from build123d import *

# Parameters (mm, degrees)
SKETCH_1_W                = 20
SKETCH_1_H                = 34
EXTRUDE_1_DEPTH           = 5
SKETCH_2_W                = 20
SKETCH_2_H                = 3
EXTRUDE_2_DEPTH           = 5
EXTRUDE_3_DEPTH           = 5
FILLET_1_R                = 3
CUT_EXTRUDE_1_DEPTH       = 2
SKETCH_7_R                = 1.6
CUT_EXTRUDE_2_DEPTH       = 41.087864079
SKETCH_8_R                = 1.75
CUT_EXTRUDE_3_DEPTH       = 41.087864079
CUT_EXTRUDE_5_DEPTH       = 3.2
SKETCH_14_W               = 10
SKETCH_14_H               = 3
EXTRUDE_26_DEPTH          = 51
SKETCH_11_W               = 51
SKETCH_11_H               = 87.152977717
SKETCH_11_R               = 11.1
SKETCH_11_R_2             = 1.6
EXTRUDE_27_DEPTH          = 5
CUT_EXTRUDE_7_DEPTH       = 3
SKETCH_16_R               = 1.6
CUT_EXTRUDE_8_DEPTH       = 89.921313531
EXTRUDE_28_DEPTH          = 6.7
SKETCH_18_W               = 40
SKETCH_18_H               = 5
CUT_EXTRUDE_9_DEPTH       = 5
CHAMFER_1_SIZE            = 2
SKETCH_19_W               = 1.7
SKETCH_19_H               = 23
EXTRUDE_31_DEPTH          = 5
SKETCH_20_W               = 5
SKETCH_20_H               = 28
EXTRUDE_33_DEPTH          = 5
EXTRUDE_34_DEPTH          = 1.7
SKETCH_24_R               = 11.1
CUT_EXTRUDE_10_DEPTH      = 1
CUT_EXTRUDE_12_DEPTH      = 88.98863563
SKETCH_26_R               = 5.1
CUT_EXTRUDE_13_DEPTH      = 89.2892972
CHAMFER_2_SIZE            = 2
EXTRUDE_35_DEPTH          = 5.7
EXTRUDE_36_DEPTH          = 2
EXTRUDE_37_DEPTH          = 26
CUT_EXTRUDE_14_DEPTH      = 91.329895384
SKETCH_32_R               = 1.6
CUT_EXTRUDE_15_DEPTH      = 89.2892972
CUT_EXTRUDE_16_DEPTH      = 10
CUT_EXTRUDE_16_DEPTH_BACK = 3.5
SKETCH_33_R               = 3


with BuildPart() as part:
    # 草图1 → 凸台-拉伸1 (new body)
    with BuildSketch(Plane.XY):
        with Locations((-10, 17)):
            Rectangle(SKETCH_1_W, SKETCH_1_H)
    extrude(amount=EXTRUDE_1_DEPTH)

    # 草图2 → 凸台-拉伸2 (add)
    with BuildSketch(Plane.XY.offset(5)):
        with Locations((-10, 32.5)):
            Rectangle(SKETCH_2_W, SKETCH_2_H)
        with Locations((-10, 1.5)):
            Rectangle(SKETCH_2_W, SKETCH_2_H)
    extrude(amount=EXTRUDE_2_DEPTH)

    # 草图4 → 凸台-拉伸3 (add)
    with BuildSketch(Plane(origin=(0, 0, 0), x_dir=(-1, 0, 0), z_dir=(0, 0, -1))):
        Polygon((0, 3), (0, 31), (-2.991740991, 31), (-20.640660029, 23.203556304), (-20.640660029, 10.796443696), (-2.991740991, 3), align=None)
        with BuildLine():
            ThreePointArc((-16, 15.25), (-17.75, 17), (-16, 18.75))
            Line((-16, 18.75), (-14, 18.75))
            ThreePointArc((-14, 18.75), (-12.25, 17), (-14, 15.25))
            Line((-14, 15.25), (-16, 15.25))
        make_face(mode=Mode.SUBTRACT)
    extrude(amount=-EXTRUDE_3_DEPTH)

    # 圆角1
    fillet_1_edges = [part.edges().sort_by_distance(p)[0] for p in [
        (20.640660029, 10.796443696, 2.5),
        (20.640660029, 23.203556304, 2.5),
    ]]
    fillet(fillet_1_edges, radius=FILLET_1_R)

    # 草图5 → 切除-拉伸1 (cut)
    with BuildSketch(Plane(origin=(0, 0, 0), x_dir=(-1, 0, 0), z_dir=(0, 0, -1))):
        with BuildLine():
            Line((-16, 20.25), (-13.505814151, 20.212208017))
            ThreePointArc((-13.505814151, 20.212208017), (-10.759461769, 16.75218561), (-14, 13.75))
            Line((-14, 13.75), (-16, 13.75))
            ThreePointArc((-16, 13.75), (-19.25, 17), (-16, 20.25))
        make_face()
    extrude(amount=-CUT_EXTRUDE_1_DEPTH, mode=Mode.SUBTRACT)

    # 草图7 → 切除-拉伸2 (cut, through all)
    with BuildSketch(Plane.XY.offset(5)):
        with Locations((-17.5, 22)):
            Circle(SKETCH_7_R)
        with Locations((-2.5, 22)):
            Circle(SKETCH_7_R)
        with Locations((-2.5, 12)):
            Circle(SKETCH_7_R)
        with Locations((-17.5, 12)):
            Circle(SKETCH_7_R)
    extrude(amount=-CUT_EXTRUDE_2_DEPTH, mode=Mode.SUBTRACT)

    # 草图8 → 切除-拉伸3 (cut, through all)
    with BuildSketch(Plane.XY.offset(5)):
        with Locations((-10, 17)):
            Circle(SKETCH_8_R)
    extrude(amount=-CUT_EXTRUDE_3_DEPTH, mode=Mode.SUBTRACT)

    # 草图9 → 切除-拉伸5 (cut)
    with BuildSketch(Plane(origin=(0, 0, 0), x_dir=(-1, 0, 0), z_dir=(0, 0, -1))):
        Polygon((11.668772273, 13.964345359), (13.463340173, 16.927371861), (11.7945679, 19.963026502), (8.331227727, 20.035654641), (6.536659827, 17.072628139), (8.2054321, 14.036973498), align=None)
    extrude(amount=-CUT_EXTRUDE_5_DEPTH, mode=Mode.SUBTRACT)

    # 草图14 → 凸台-拉伸26 (add)
    with BuildSketch(Plane.ZY.offset(20)):
        with Locations((5, 32.5)):
            Rectangle(SKETCH_14_W, SKETCH_14_H)
    extrude(amount=EXTRUDE_26_DEPTH)

    # 草图11 → 凸台-拉伸27 (add)
    with BuildSketch(Plane.XZ.offset(-31)):
        with Locations((-45.5, 1.423511141)):
            Rectangle(SKETCH_11_W, SKETCH_11_H)
        with Locations(Location((-48, 22, 0), (0, 0, 270))):
            Circle(SKETCH_11_R, mode=Mode.SUBTRACT)
        with Locations(Location((-32.5, 37.5, 0), (0, 0, 270))):
            Circle(SKETCH_11_R_2, mode=Mode.SUBTRACT)
        with Locations(Location((-32.5, 6.5, 0), (0, 0, 90))):
            Circle(SKETCH_11_R_2, mode=Mode.SUBTRACT)
        with Locations(Location((-63.5, 6.5, 0), (0, 0, 270))):
            Circle(SKETCH_11_R_2, mode=Mode.SUBTRACT)
        with Locations(Location((-63.5, 37.5, 0), (0, 0, 90))):
            Circle(SKETCH_11_R_2, mode=Mode.SUBTRACT)
    extrude(amount=EXTRUDE_27_DEPTH)

    # 草图15 → 切除-拉伸7 (cut)
    with BuildSketch(Plane.XZ.offset(-26)):
        Polygon((-67.3, 43.3), (-28.7, 43.3), (-26.7, 41.3), (-26.7, 2.7), (-28.7, 0.7), (-67.3, 0.7), (-69.3, 2.7), (-69.3, 41.3), align=None)
    extrude(amount=-CUT_EXTRUDE_7_DEPTH, mode=Mode.SUBTRACT)

    # 草图16 → 切除-拉伸8 (cut, through all)
    with BuildSketch(Plane.XZ.offset(-29)):
        with Locations(Location((-63.5, 6.5, 0), (0, 0, 90))):
            Circle(SKETCH_16_R)
        with Locations(Location((-32.5, 6.5, 0), (0, 0, 90))):
            Circle(SKETCH_16_R)
    extrude(amount=-CUT_EXTRUDE_8_DEPTH, mode=Mode.SUBTRACT)

    # 草图17 → 凸台-拉伸28 (add)
    with BuildSketch(Plane.ZY.offset(20)):
        Polygon((0, 26), (5, 26), (5, 3), (10, 3), (10, 0), (0, 0), align=None)
    extrude(amount=EXTRUDE_28_DEPTH)

    # 草图18 → 切除-拉伸9 (cut)
    with BuildSketch(Plane(origin=(-20, 0, 0), x_dir=(0, 0, -1), z_dir=(1, 0, 0))):
        with Locations((-25, 28.5)):
            Rectangle(SKETCH_18_W, SKETCH_18_H)
    extrude(amount=-CUT_EXTRUDE_9_DEPTH, mode=Mode.SUBTRACT)

    # 倒角1
    chamfer_1_edges = [part.edges().sort_by_distance(p)[0] for p in [
        (-71, 34, 5),
        (-71, 28.5, 45),
        (-25, 28.5, 45),
    ]]
    chamfer(chamfer_1_edges, length=CHAMFER_1_SIZE)

    # 草图19 → 凸台-拉伸31 (add)
    with BuildSketch(Plane.XY.offset(5)):
        with Locations((-25.85, 14.5)):
            Rectangle(SKETCH_19_W, SKETCH_19_H)
    extrude(amount=EXTRUDE_31_DEPTH)

    # 草图20 → 凸台-拉伸33 (add)
    with BuildSketch(Plane(origin=(-25, 0, 0), x_dir=(0, 0, -1), z_dir=(1, 0, 0))):
        with Locations((-7.5, 17)):
            Rectangle(SKETCH_20_W, SKETCH_20_H)
    extrude(amount=EXTRUDE_33_DEPTH)

    # 草图23 → 凸台-拉伸34 (add)
    with BuildSketch(Plane(origin=(-25, 0, 0), x_dir=(0, 0, -1), z_dir=(1, 0, 0))):
        Polygon((-10, 0), (-10, 26), (-36, 26), align=None)
    extrude(amount=-EXTRUDE_34_DEPTH)

    # 草图24 → 切除-拉伸10 (cut)
    with BuildSketch(Plane.XZ.offset(-26)):
        with Locations(Location((-46, -20, 0), (0, 0, 270))):
            Circle(SKETCH_24_R)
    extrude(amount=-CUT_EXTRUDE_10_DEPTH, mode=Mode.SUBTRACT)

    # 草图25 → 切除-拉伸12 (cut, through all)
    with BuildSketch(Plane.XZ.offset(-26)):
        with BuildLine():
            Line((-78.519072423, -1.3), (-59, -1.3))
            Line((-59, -1.3), (-59, -20))
            ThreePointArc((-59, -20), (-51.523309234, -31.768307232), (-37.693376137, -30))
            Line((-37.693376137, -30), (-21, -30))
            Line((-21, -30), (-21, 0))
            Line((-21, 0), (-16.887627511, 0))
            Line((-16.887627511, 0), (-16.887627511, -53.680594447))
            Line((-16.887627511, -53.680594447), (-78.519072423, -54.78523931))
            Line((-78.519072423, -54.78523931), (-78.519072423, -1.3))
        make_face()
    extrude(amount=-CUT_EXTRUDE_12_DEPTH, mode=Mode.SUBTRACT)

    # 草图26 → 切除-拉伸13 (cut, through all)
    with BuildSketch(Plane.XZ.offset(-27)):
        with Locations(Location((-46, -20, 0), (0, 0, 270))):
            Circle(SKETCH_26_R)
    extrude(amount=-CUT_EXTRUDE_13_DEPTH, mode=Mode.SUBTRACT)

    # 倒角2
    chamfer_2_edges = [part.edges().sort_by_distance(p)[0] for p in [
        (-71, 28.5, -1.3),
    ]]
    chamfer(chamfer_2_edges, length=CHAMFER_2_SIZE)

    # 草图27 → 凸台-拉伸35 (add)
    with BuildSketch(Plane.ZY.offset(26.7)):
        Polygon((0, 0), (0, 26), (-30, 26), (-1.72204929, 0), align=None)
    extrude(amount=-EXTRUDE_35_DEPTH)

    # 草图28 → 凸台-拉伸36 (add)
    with BuildSketch(Plane.XY.offset(0.7)):
        Polygon((-55.07905283, 26), (-26.7, 26), (-26.7, 0), align=None)
    extrude(amount=-EXTRUDE_36_DEPTH)

    # 草图29 → 凸台-拉伸37 (add)
    with BuildSketch(Plane.XZ.offset(-26)):
        Polygon((-26.7, 2.7), (-28.7, 0.7), (-26.7, 0.7), align=None)
    extrude(amount=EXTRUDE_37_DEPTH)

    # 草图30 → 切除-拉伸14 (cut, through all)
    with BuildSketch(Plane(origin=(0, 0, 0.7), x_dir=(-1, 0, 0), z_dir=(0, 0, -1))):
        Polygon((28.7, 0), (26.7, 0), (28.7, 1.832337404), align=None)
    extrude(amount=-CUT_EXTRUDE_14_DEPTH, mode=Mode.SUBTRACT)

    # 草图32 → 切除-拉伸15 (cut, through all)
    with BuildSketch(Plane.XZ.offset(-27)):
        with Locations(Location((-46, -12, 0), (0, 0, 270))):
            Circle(SKETCH_32_R)
        with Locations(Location((-54, -20, 0), (0, 0, 270))):
            Circle(SKETCH_32_R)
        with Locations(Location((-38, -20, 0), (0, 0, 270))):
            Circle(SKETCH_32_R)
        with Locations(Location((-46, -28, 0), (0, 0, 270))):
            Circle(SKETCH_32_R)
    extrude(amount=-CUT_EXTRUDE_15_DEPTH, mode=Mode.SUBTRACT)

    # 草图33 → 切除-拉伸16 (cut, two sides: drawn at the far end of the back side and taken through both)
    with BuildSketch(Plane.XY.offset(5).offset(-CUT_EXTRUDE_16_DEPTH_BACK)):
        with Locations((-2.5, 12)):
            Circle(SKETCH_33_R)
        with Locations(Location((-17.5, 12, 0), (0, 0, 213.557309762))):
            Circle(SKETCH_33_R)
        with Locations((-2.5, 22)):
            Circle(SKETCH_33_R)
        with Locations(Location((-17.5, 22, 0), (0, 0, 146.442690238))):
            Circle(SKETCH_33_R)
    extrude(amount=CUT_EXTRUDE_16_DEPTH + CUT_EXTRUDE_16_DEPTH_BACK, mode=Mode.SUBTRACT)


solid = part.part
Build history of the part. All positions in model axes, mm. A direction names the side the tool comes from. Give positions to 0.01 mm unless a question says otherwise; leave off trailing zeros. Order: outer loops, then holes, each group sorted by start corner. A loop starts at its lowest first (then second) coordinate and runs counter-clockwise, first axis right, second up. Notation, with made-up numbers: M 43.25,58 L 56.25,58 A24 ccw 56.25,73 Z; hole C 83,-0.5 d5. An arc over 180 degrees is marked long. Put each result on its own line as item: value.
Item 1: Drop flat-ended pins along their axis: pin 1 Ø8 at (x, y) = (8.5, 23) entering from +Z; pin 2 Ø2.5 at (x, y) = (-17.5, 12) entering from -Z; pin 3 Ø1 at (x, z) = (-36.5, -19.5) entering from -Y; pin 4 Ø1.5 at (x, y) = (-42, 29.5) entering from -Z. Give the stop position or say it passes through.
Results are:
pin 1: z = 5
pin 2: through
pin 3: y = 27
pin 4: z = -32.59
Item 2: Wall check: probe 1 along X at (y, z) = (30, 6); probe 2 along X at (y, z) = (12, 3.55); probe 3 along Z at (x, y) = (10, 22). Give the ranges that are in metal, low to high.
Results are:
probe 1: -71 to -65.02, -61.98 to -34.02, -30.98 to -20
probe 2: -26.7 to -20.5, -14.5 to -5.5, 0.5 to 20.55
probe 3: 0 to 5
Item 3: Pull direction Z, two halves, no side cores. Call faces 5 (the face through (-48, 27, 43.3)), 6 (the face through (19.25, 16.93, 0.99)), 7 (the face through (-26, 13, 23)), 8 (the face through (-11.5, 15.7, 3.2)): +Z half, -Z half, draft (parallel to the pull), parting line (faces both ways), or undercut.
Results are:
face 5: undercut
face 6: draft
face 7: +Z half
face 8: -Z half
Item 4: Cut at D-D on z = 37.5. Write the cut outline in (x, y).
Results are:
outline: M -71,26 L -69.3,26 L -69.3,29 L -65.1,29 L -65.1,31 L -71,31 Z; M -61.9,29 L -34.1,29 L -34.1,31 L -61.9,31 Z; M -30.9,29 L -26.7,29 L -26.7,26 L -25,26 L -25,31 L -30.9,31 Z
Item 5: Cut at B-B on z = 6.5. Write the cut outline in (x, y).
Results are:
outline: M -71,26 L -69.3,26 L -69.3,29 L -65.1,29 L -65.1,34 L -69,34 L -71,32 Z; M -61.9,29 L -34.1,29 L -34.1,34 L -61.9,34 Z; M -30.9,29 L -26.7,29 L -26.7,0 L 0,0 L 0,3 L -20,3 L -20,10.34 A3 cw -20,13.66 L -20,20.34 A3 cw -20,23.66 L -20,31 L 0,31 L 0,34 L -30.9,34 Z
Item 6: Which spindle directions (+Z, -Z, +X, -X, +Y, -Y) get a long thin tool onto all of the face, cutting with end or side? Do faces 1 (the face through (-12.641, 18.424, 1.578)), 2 (the face through (17.75, 16.96, 3.48)), 3 (the face through (-20.1, 13.5, 3.8)), 4 (the face through (-27.7, 27.5, 42.3)). Say none if no direction does.
Results are:
face 1: -Z
face 2: +Z, -Z
face 3: +Z
face 4: -Y
Item 7: Cut at C-C on z = -12. Write the cut outline in (x, y).
Results are:
outline: M -59,26 L -53.69,26 L -53.69,27 L -47.6,27 L -47.6,31 L -59,31 Z; M -44.4,27 L -38.31,27 L -38.31,26 L -26.7,26 L -26.7,9.45 L -21,9.45 L -21,31 L -44.4,31 Z
Item 8: Cut at A-A on x = -17.5. Write the cut outline in (y, z), then the cut area to 3 significant figures.
Results are:
outline: M 0,0 L 10.4,0 L 10.4,1.5 L 9,1.5 L 9,5 L 3,5 L 3,10 L 0,10 Z; M 13.6,0 L 20.4,0 L 20.4,1.5 L 19,1.5 L 19,5 L 15,5 L 15,1.5 L 13.6,1.5 Z; M 23.6,0 L 34,0 L 34,10 L 31,10 L 31,5 L 25,5 L 25,1.5 L 23.6,1.5 Z
area: 148 mm2
